Input: part model. Units: mm. Frame: model coordinates. A direction names the side the tool comes from. Give positions to 0.01 mm unless a question says otherwise; leave off trailing zeros. Loops run counter-clockwise (first coordinate to the right, second up) from the corner with the lowest first, then second, coordinate; pieces in that order, holes last. Notation, with made-up numbers: (68.25, -19) -> (84.25, -19) arc R10 ccw to (84.25, -5) -> close; hole circle Ø1 at (5.25, 4). An arc over 180 degrees is marked (long way). One line per question, with ' | ' between items.
from build123d import *

# Parameters (mm, degrees)
BOSS_EXTRUDE1_DEPTH = 40
BOSS_EXTRUDE2_START = 35
BOSS_EXTRUDE2_DEPTH = 5
BOSS_EXTRUDE3_START = -30
BOSS_EXTRUDE3_DEPTH = 5
SKETCH2_R           = 2.5
CUT_EXTRUDE1_DEPTH  = 15
BOSS_EXTRUDE4_START = 2.5
SKETCH4_R           = 2.5
BOSS_EXTRUDE4_DEPTH = 5
BOSS_EXTRUDE5_START = -7.5
SKETCH4_2_R         = 2.5
BOSS_EXTRUDE5_DEPTH = 5
FILLET1_R           = 1
FILLET2_R           = 2.5


with BuildPart() as part:
    # Sketch1 → Boss-Extrude1 (new, symmetric)
    with BuildSketch(Plane.XY):
        with BuildLine():
            Line((-11, 24), (-11.5, 24))
            Line((-11.5, 24), (-11.5, 15.5))
            Line((-11.5, 15.5), (-11, 15.5))
            Line((-11, 15.5), (-11, 10.198039027))
            ThreePointArc((-11, 10.198039027), (-6.625817064, -13.457286065), (14.790199458, -2.5))
            Line((14.790199458, -2.5), (9.682458366, -2.5))
            ThreePointArc((9.682458366, -2.5), (-10, 0), (9.682458366, 2.5))
            Line((9.682458366, 2.5), (14.790199458, 2.5))
            ThreePointArc((14.790199458, 2.5), (8.269504868, 12.514603039), (-3.5, 14.585952146))
            Line((-3.5, 14.585952146), (-3.5, 24))
            Line((-3.5, 24), (-11, 24))
        make_face()
    extrude(amount=BOSS_EXTRUDE1_DEPTH, both=True)

    # Sketch1_3 → Boss-Extrude2 (add)
    with BuildSketch(Plane.XY.offset(BOSS_EXTRUDE2_START)):
        with BuildLine():
            Line((10.325172425, 10.880754312), (-3.5, 24))
            Line((-3.5, 24), (-3.5, 14.585952146))
            ThreePointArc((-3.5, 14.585952146), (3.883022973, 14.488689816), (10.325172425, 10.880754312))
        make_face()
    extrude(amount=-BOSS_EXTRUDE2_DEPTH)

    # Sketch1_4 → Boss-Extrude3 (add)
    with BuildSketch(Plane.XY.offset(BOSS_EXTRUDE3_START)):
        with BuildLine():
            Line((10.325172425, 10.880754312), (-3.5, 24))
            Line((-3.5, 24), (-3.5, 14.585952146))
            ThreePointArc((-3.5, 14.585952146), (3.883022973, 14.488689816), (10.325172425, 10.880754312))
        make_face()
    extrude(amount=-BOSS_EXTRUDE3_DEPTH)

    # Sketch2 → Cut-Extrude1 (cut)
    with BuildSketch(Plane(origin=(0, 0, 0), x_dir=(0, 0, -1), z_dir=(1, 0, 0))):
        with Locations((-25, 19.292976073)):
            Circle(SKETCH2_R)
        with Locations((25, 19.292976073)):
            Circle(SKETCH2_R)
    extrude(amount=-CUT_EXTRUDE1_DEPTH, mode=Mode.SUBTRACT)

    # Sketch4 → Boss-Extrude4 (add)
    # profile 1 of 2: a face of its own
    with BuildSketch(Plane(origin=(0, 0, 0), x_dir=(1, 0, 0), z_dir=(0, 1, 0)).offset(BOSS_EXTRUDE4_START)):
        with BuildLine():
            Line((17.290199458, 21.25), (12.290199458, 21.25))
            Line((12.290199458, 21.25), (12.290199458, 28.75))
            Line((12.290199458, 28.75), (17.290199458, 28.75))
            ThreePointArc((17.290199458, 28.75), (21.040199458, 25), (17.290199458, 21.25))
        make_face()
        with Locations(Location((17.290199458, 25, 0), (0, 0, 270))):
            Circle(SKETCH4_R, mode=Mode.SUBTRACT)
    # profile 2 of 2: a face of its own
    with BuildSketch(Plane(origin=(0, 0, 0), x_dir=(1, 0, 0), z_dir=(0, 1, 0)).offset(BOSS_EXTRUDE4_START)):
        with BuildLine():
            Line((12.290199458, -28.75), (17.290199458, -28.75))
            ThreePointArc((17.290199458, -28.75), (21.040199458, -25), (17.290199458, -21.25))
            Line((17.290199458, -21.25), (12.290199458, -21.25))
            Line((12.290199458, -21.25), (12.290199458, -28.75))
        make_face()
        with Locations(Location((17.290199458, -25, 0), (0, 0, 90))):
            Circle(SKETCH4_R, mode=Mode.SUBTRACT)
    extrude(amount=BOSS_EXTRUDE4_DEPTH)

    # Sketch4_2 → Boss-Extrude5 (add)
    # profile 1 of 2: a face of its own
    with BuildSketch(Plane(origin=(0, 0, 0), x_dir=(1, 0, 0), z_dir=(0, 1, 0)).offset(BOSS_EXTRUDE5_START)):
        with BuildLine():
            Line((17.290199458, 21.25), (12.290199458, 21.25))
            Line((12.290199458, 21.25), (12.290199458, 28.75))
            Line((12.290199458, 28.75), (17.290199458, 28.75))
            ThreePointArc((17.290199458, 28.75), (21.040199458, 25), (17.290199458, 21.25))
        make_face()
        with Locations(Location((17.290199458, 25, 0), (0, 0, 270))):
            Circle(SKETCH4_2_R, mode=Mode.SUBTRACT)
    # profile 2 of 2: a face of its own
    with BuildSketch(Plane(origin=(0, 0, 0), x_dir=(1, 0, 0), z_dir=(0, 1, 0)).offset(BOSS_EXTRUDE5_START)):
        with BuildLine():
            Line((12.290199458, -28.75), (17.290199458, -28.75))
            ThreePointArc((17.290199458, -28.75), (21.040199458, -25), (17.290199458, -21.25))
            Line((17.290199458, -21.25), (12.290199458, -21.25))
            Line((12.290199458, -21.25), (12.290199458, -28.75))
        make_face()
        with Locations(Location((17.290199458, -25, 0), (0, 0, 90))):
            Circle(SKETCH4_2_R, mode=Mode.SUBTRACT)
    extrude(amount=BOSS_EXTRUDE5_DEPTH)

    # Fillet1
    fillet1_edges = [part.edges().sort_by_distance(p)[0] for p in [
        (14.113474534, -5.080338234, -21.25),
        (14.113474534, -5.080338234, -28.75),
        (14.113474534, -5.080338234, 21.25),
        (14.113474534, -5.080338234, 28.75),
        (14.113474534, 5.080338234, -28.75),
        (14.113474534, 5.080338234, -21.25),
        (14.113474534, 5.080338234, 28.75),
        (14.113474534, 5.080338234, 21.25),
    ]]
    fillet(fillet1_edges, radius=FILLET1_R)

    # Fillet2
    fillet2_edges = [part.edges().sort_by_distance(p)[0] for p in [
        (-7.5, 24, -40),
        (-7.5, 24, 40),
    ]]
    fillet(fillet2_edges, radius=FILLET2_R)


solid = part.part
1. Section query B-B (x = -9). Output: boundary loops of the cut face in (y, z), then the cut area to 3 significant figures.
Determined:
outline: (-12, -40) -> (-4.36, -40) -> (-4.36, 40) -> (-12, 40) -> close; (4.36, -40) -> (21.5, -40) arc R2.5 ccw to (24, -37.5) -> (24, 37.5) arc R2.5 ccw to (21.5, 40) -> (4.36, 40) -> close; hole circle Ø5 at (19.29, -25); hole circle Ø5 at (19.29, 25) | area: 2,140 mm2
2. Reachability of faces 1 (the flat face through (13, 2.5, -1)), 2 (the flat face through (16, 6, -28.75)), 3 (the flat face through (16, 6, 21.25)), 4 (the flat face through (14, 7.5, -25)) from +Z, -Z, +X, -X, +Y, -Y: full face, straight path, thin tool, end or side. Return the list, or none.
Determined:
face 1: +Z, -Z, +X | face 2: -Z, +X, +Y | face 3: +X, +Y | face 4: +Z, -Z, +X, +Y
3. Section query D-D (x = -1.5). Output: boundary loops of the cut face in (y, z).
Determined:
outline: (-14.92, -40) -> (-9.89, -40) -> (-9.89, 40) -> (-14.92, 40) -> close; (9.89, -40) -> (14.92, -40) -> (14.92, -35) -> (22.1, -35) -> (22.1, -30) -> (14.92, -30) -> (14.92, 30) -> (22.1, 30) -> (22.1, 35) -> (14.92, 35) -> (14.92, 40) -> (9.89, 40) -> close
4. Section query A-A (z = 25). Output: boundary loops of the cut face in (x, y), then the cut area to 3 significant figures.
Determined:
outline: (-11.5, 15.5) -> (-11, 15.5) -> (-11, 10.2) arc R15 ccw (long way) to (12.99, -7.5) -> (14.79, -7.5) -> (14.79, -2.5) -> (9.68, -2.5) arc R10 cw (long way) to (9.68, 2.5) -> (14.79, 2.5) -> (14.79, 7.5) -> (12.99, 7.5) arc R15 ccw to (-3.5, 14.59) -> (-3.5, 16.79) -> (-11.5, 16.79) -> close; (-11.5, 21.79) -> (-3.5, 21.79) -> (-3.5, 24) -> (-11.5, 24) -> close; (19.79, -7.5) -> (21.04, -7.5) -> (21.04, -2.5) -> (19.79, -2.5) -> close; (19.79, 2.5) -> (21.04, 2.5) -> (21.04, 7.5) -> (19.79, 7.5) -> close | area: 435 mm2
5. Pull-direction query (Y, two-part tool) for faces 5 (the cylindrical face through (15.769, 4.965, -26.984)), 6 (the flat face through (-11, 13, 1)), 7 (the flat face through (3.51, 17.35, -32.47)); classes: pulls with the +Y half, pulls with the -Y half, needs draft (parallel to the pull), parting line crosses it, or undercut.
Determined:
face 5: needs draft | face 6: undercut | face 7: pulls with the +Y half
6. Pin query (flat end, axial travel): P1, Ø8, axis at x = 17.29, z = 25, coming from the +Y side; P2, Ø0.9, axis at x = 15.5, y = -5, coming from the -Z side; P3, Ø5, axis at x = -5, z = 27.5, coming from the -Y side. Return the tip coordinate at first contact, or that it passes through.
Determined:
P1: stops at y = 7.5 | P2: stops at z = -28.76 | P3: stops at y = -14.79
7. Section query C-C (z = -17.5). Output: boundary loops of the cut face in (x, y).
Determined:
outline: (-11.5, 15.5) -> (-11, 15.5) -> (-11, 10.2) arc R15 ccw (long way) to (14.79, -2.5) -> (9.68, -2.5) arc R10 cw (long way) to (9.68, 2.5) -> (14.79, 2.5) arc R15 ccw to (-3.5, 14.59) -> (-3.5, 24) -> (-11.5, 24) -> close
8. Ray query, line 1 along Y through (x, z) = (-8.5, 25); line 2 along X through (y, z) = (5.15, -25); line 3 along Z through (x, y) = (1, 16). Return the intervals inside material, ascending. Write a range as from..to.
Determined:
line 1: y = -12.36..-5.27, 5.27..16.79, 21.79..24 | line 2: x = -14.09..-8.57, 8.57..14.79, 19.79..21.04 | line 3: z = -35..-30, 30..35
